Print and shaded views of the part. All mm, measured from the part's lowest x, y and z. Coordinates: 2 decimals unless noted, no trailing zeros. Loops run counter-clockwise (first coordinate to the right, second up) from the corner with the lowest first, then second, coordinate; pieces in that order, holes last.
1) Pin check, flat tips, straight feed: pin 1 Ø3 at (y, z) = (12, 203) entering from -X; pin 2 Ø9.5 at (y, z) = (11.5, 16.5) entering from +X; pin 3 Ø9.5 at (x, y) = (11, 11) entering from +Z; pin 4 Ø5 at (x, z) = (204.5, 312.5) entering from -Y. Stop position of each tip, or through.
2) Saw through at A-A, the plane y = 13.5. Write the cut outline in (x, z).
3) Saw through at B-B, the plane z = 30. Write the cut outline in (x, y), and give its area (3 significant figures).
4) Wall check: line 1 along X through (y, z) = (15.75, 188). Give the ranges that are in metal, low to high.
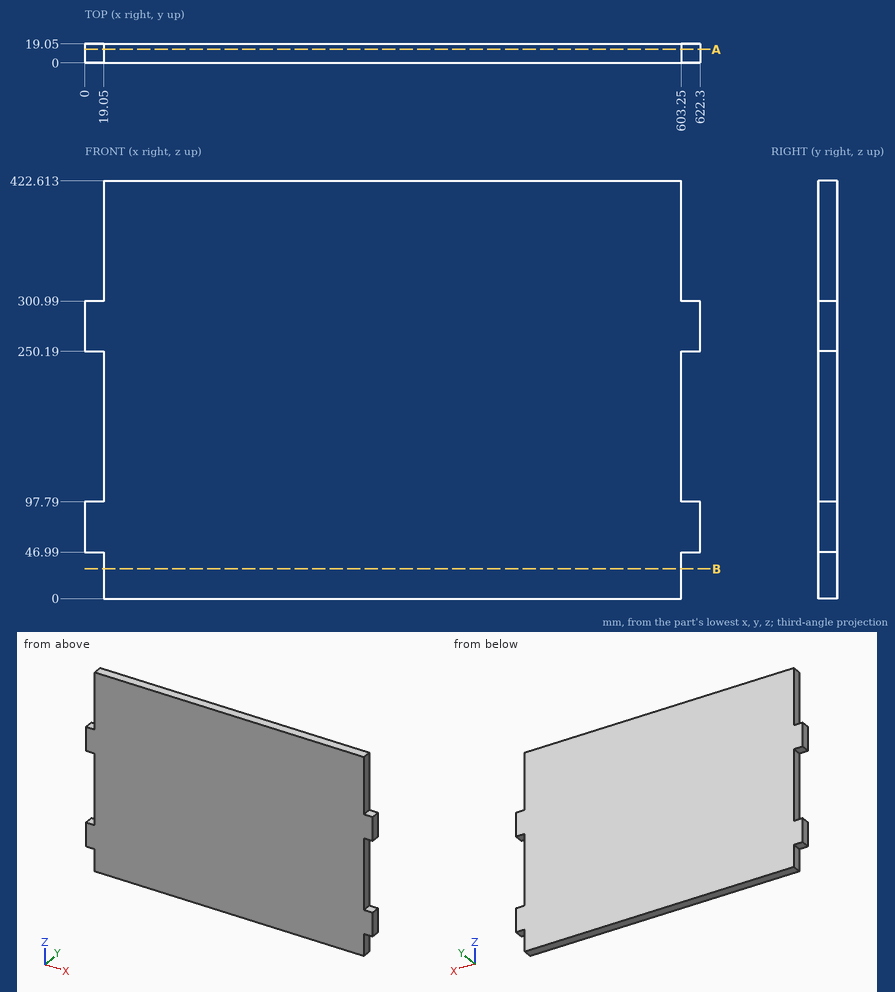
Data:
1. pin 1: stops at x = 19.05
1. pin 2: stops at x = 603.25
1. pin 3: stops at z = 300.99
1. pin 4: stops at y = 0
2. outline: (0, 46.99) - (19.05, 46.99) - (19.05, 0) - (603.25, 0) - (603.25, 46.99) - (622.3, 46.99) - (622.3, 97.79) - (603.25, 97.79) - (603.25, 250.19) - (622.3, 250.19) - (622.3, 300.99) - (603.25, 300.99) - (603.25, 422.61) - (19.05, 422.61) - (19.05, 300.99) - (0, 300.99) - (0, 250.19) - (19.05, 250.19) - (19.05, 97.79) - (0, 97.79) - close
3. outline: (19.05, 0) - (603.25, 0) - (603.25, 19.05) - (19.05, 19.05) - close
3. area: 11,100 mm2
4. line 1: x = 19.05 to 603.25
